```python
from build123d import *

# Parameters (mm, degrees)
F1_DEPTH = 25.4
F2_DEPTH = 6.35
F0_R     = 6.35
F3_DEPTH = 12.7


with BuildPart() as f1:
    # F0 (on Front) → F1 (new body)
    with BuildSketch(Plane.XZ):
        with BuildLine():
            ThreePointArc((-25.623486, -23.949636), (-13.346651, -14.667498), (-8.683683, 0))
            ThreePointArc((-8.683683, 0), (-13.346651, 14.667498), (-25.623486, 23.949636))
            ThreePointArc((-25.623486, 23.949636), (-59.483683, 0), (-25.623486, -23.949636))
        make_face()
        with BuildLine():
            ThreePointArc((-31.31444, 12.394406), (-24.172594, 7.941052), (-21.383683, 0))
            ThreePointArc((-21.383683, 0), (-42.205979, -9.763109), (-36.39444, 12.48801))
            Line((-36.39444, 12.48801), (-36.39444, 15.597617))
            Line((-36.39444, 15.597617), (-31.31444, 15.597617))
            Line((-31.31444, 15.597617), (-31.31444, 12.394406))
        make_face(mode=Mode.SUBTRACT)
    extrude(amount=F1_DEPTH)

    # F0 (on Front) → F2 (join)
    with BuildSketch(Plane.XZ):
        with BuildLine():
            ThreePointArc((-25.623486, 23.949636), (-13.346651, 14.667498), (-8.683683, 0))
            ThreePointArc((-8.683683, 0), (-13.346651, -14.667498), (-25.623486, -23.949636))
            Line((-25.623486, -23.949636), (29.342367, -12.429951))
            ThreePointArc((29.342367, -12.429951), (14.037311, 0), (29.342367, 12.429951))
            Line((29.342367, 12.429951), (-25.623486, 23.949636))
        make_face()
    extrude(amount=F2_DEPTH)

    # F0 (on Front) → F3 (join)
    with BuildSketch(Plane.XZ):
        with BuildLine():
            ThreePointArc((39.437311, 0), (36.595664, 8.006428), (29.342367, 12.429951))
            ThreePointArc((29.342367, 12.429951), (14.037311, 0), (29.342367, -12.429951))
            ThreePointArc((29.342367, -12.429951), (36.595664, -8.006428), (39.437311, 0))
        make_face()
        with Locations((26.737311, 0)):
            Circle(F0_R, mode=Mode.SUBTRACT)
    extrude(amount=F3_DEPTH)


solid = f1.part
```
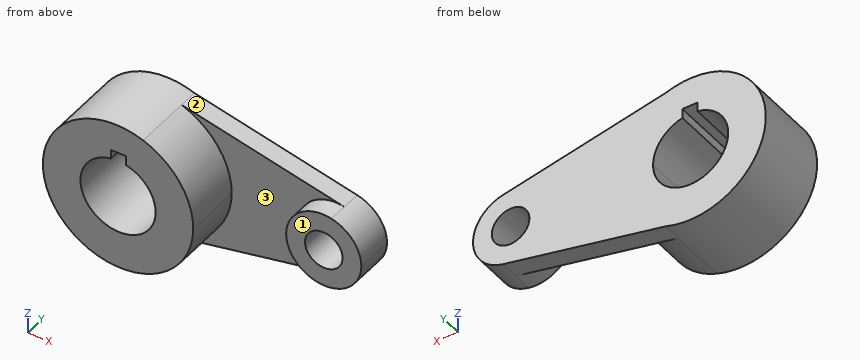
The listing builds one solid part. Answer for the finished solid, in the listing's coordinates (mm). Face numbers are marked on the shaded views. Round coordinates to 2 decimals unless told otherwise and drop trailing zeros. Loops run counter-clockwise (first coordinate to the right, second up) from the corner with the lowest first, then second, coordinate; pieces in that order, holes last.
1) A cutting plane is placed at A-A on y = -10. Determine the outline of the cut face in (x, z).
Outcome:
outline: circle Ø50.8 at (-34.08, 0); (29.34, -12.43) arc R12.7 ccw to (39.44, 0) arc R12.7 ccw to (29.34, 12.43) arc R12.7 ccw (long way) to start; hole (-36.39, 12.49) arc R12.7 ccw (long way) to (-21.38, 0) arc R12.7 ccw to (-31.31, 12.39) - (-31.31, 15.6) - (-36.39, 15.6) - close; hole circle Ø12.7 at (26.74, 0)
2) A cutting plane is placed at D-D on x = -34.5. Determine the outline of the cut face in (y, z).
Outcome:
outline: (-25.4, -25.4) - (0, -25.4) - (0, -12.69) - (-25.4, -12.69) - close; (-25.4, 15.6) - (0, 15.6) - (0, 25.4) - (-25.4, 25.4) - close
3) A cutting plane is placed at B-B on y = -23.25. Determine the outline of the cut face in (x, z), plus the area to 3 significant figures.
Outcome:
outline: circle Ø50.8 at (-34.08, 0); hole (-36.39, 12.49) arc R12.7 ccw (long way) to (-21.38, 0) arc R12.7 ccw to (-31.31, 12.39) - (-31.31, 15.6) - (-36.39, 15.6) - close
area: 1,500 mm2
4) For a pull along X with two mould halves and no side action, classify the marked faces 1, 2 and 3 as released by +X, released by -X, zero draft, split by the parting line, or undercut.
Outcome:
face 1: zero draft
face 2: released by +X
face 3: undercut
5) A cutting plane is placed at C-C on z = -4. Determine the outline of the cut face in (x, y).
Outcome:
outline: (-59.17, -25.4) - (-46.14, -25.4) - (-46.14, 0) - (-59.17, 0) - close; (-22.03, -25.4) - (-9, -25.4) - (-9, -6.35) - (14.68, -6.35) - (14.68, -12.7) - (21.81, -12.7) - (21.81, 0) - (-22.03, 0) - close; (31.67, -12.7) - (38.79, -12.7) - (38.79, 0) - (31.67, 0) - close
6) Consider line 1 (Z direction, x = -34.5, y = -17.75); line 2 (Z direction, x = 30.5, y = -4.5); line 3 (Y direction, x = 24, z = -11). Determine where each line is inside the solid, lowest interval first.
Outcome:
line 1: z = -25.4 to -12.69, 15.6 to 25.4
line 2: z = -12.13 to -5.12, 5.12 to 12.13
line 3: y = -12.7 to 0
7) Given P1, Ø2, axis at x = -45, z = -14.5, coming from the +Y side; P2, Ø1.5, axis at y = -18, z = 13.5, coming from the +X side; P3, Ø3, axis at y = -19.5, z = -5, coming from the -X side; P4, Ø14.5, axis at x = 0.5, z = -1, coming from the -Y side, each flat-ended and moving along its own axis, determine where each tip first touches the part or whether it passes through.
Outcome:
P1: stops at y = 0
P2: stops at x = -12.12
P3: stops at x = -59.24
P4: stops at y = -6.35
